Part model, mm, in its own coordinate system. Coordinates: 2 decimals unless noted, no trailing zeros. Write each loop counter-clockwise with the first axis right and the second up, starting at its lowest first coordinate (ties: lowest second). Pieces come first, ordered by that corner, then holes. Notation, with made-up numbers: (22, 30.5) -> (31, 30.5) arc R8 cw to (31, 45.5) -> close; hole circle Ø6 at (30.25, -2.5). An arc over 180 degrees is marked (long way). Write item = value, one per line.
from build123d import *

# Parameters (mm, degrees)
F1_DEPTH = 25
F2_SIZE  = 8


with BuildPart() as f1:
    # F0 (on Front) → F1 (new body)
    with BuildSketch(Plane.XZ):
        with BuildLine():
            ThreePointArc((54.215298, -140.742492), (47.354384, -73.095896), (49.734695, -5.143939))
            ThreePointArc((49.734695, -5.143939), (7.576454, 49.42264), (-48.991684, 9.990741))
            ThreePointArc((-48.991684, 9.990741), (-58.804788, -73.485486), (-54.496368, -157.42603))
            ThreePointArc((-54.496368, -157.42603), (8.342952, -204.363546), (54.215298, -140.742492))
        make_face()
    extrude(amount=F1_DEPTH)

    # F2
    f2_edges = [f1.edges().sort_by_distance(p)[0] for p in [
        (7.576454, -25, 49.42264),
    ]]
    chamfer(f2_edges, length=F2_SIZE)


solid = f1.part
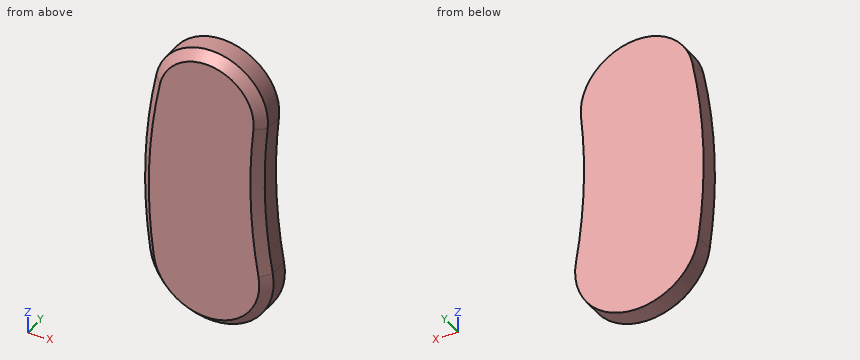
Q1. Pin check, flat tips, straight feed: pin 1 (3 mm diameter, centred on y = -3, z = -39.5, fed in from -X); pin 2 (12 mm diameter, centred on x = -43.5, y = -6, fed in from +Z); pin 3 (6 mm diameter, centred on y = -21, z = -102, fed in from +X). Stop position of each tip, or through.
Model answer:
pin_1 = -56.68
pin_2 = 33.07
pin_3 = 48.16
Q2. Probe line 1 (Z direction, x = 1, y = -2.5); line 2 (Z direction, x = -35, y = -8.75); line 3 (X direction, y = -20.5, z = -21). List the from-to ranges inside material, lowest first. Write a range as from..to.
Model answer:
line_1 = -204.99..49.99
line_2 = -192.43..35.71
line_3 = -50.77..44.84
Q3. Saw through at A-A on y = -19.5. Give the cut face in (x, z), and give its area (3 significant figures).
Model answer:
outline = (-52.02, -157.09) arc R52.5 ccw (long way) to (51.75, -141.16) arc R502.5 cw to (47.25, -4.89) arc R47.5 ccw to (-46.54, 9.49) arc R497.5 ccw to start
area = 23,100 mm²
